The listing builds one solid part. Answer for the finished solid, in the listing's coordinates (mm). Coordinates: 2 decimals unless noted, no trailing zeros. Order: outer loops, then holes, each group sorted by start corner. A loop starts at its lowest first (then second) coordinate and runs counter-clockwise, first axis right, second up. Notation, with made-up numbers: (1.5, 82.5) -> (6.5, 82.5) arc R27 ccw to (6.5, 120.5) -> close; hole circle Ø1 at (-23.5, 41.5). An arc over 180 degrees is marked (long way). Write item = value, one per line. Start each with the question number.
```python
from build123d import *

# Parameters (mm, degrees)
SKETCH_1_R          = 60
EXTRUDE_1_DEPTH     = 2
SKETCH_2_R          = 4
CUT_EXTRUDE_1_DEPTH = 2


with BuildPart() as part:
    # 草图1 → 凸台-拉伸1 (new body)
    with BuildSketch(Plane(origin=(0, 0, 0), x_dir=(1, 0, 0), z_dir=(0, 1, 0))):
        with Locations(Location((0, 0, 0), (0, 0, 270))):
            Circle(SKETCH_1_R)
    extrude(amount=EXTRUDE_1_DEPTH)

    # 草图2 → 切除-拉伸1 (cut)
    with BuildSketch(Plane(origin=(0, 2, 0), x_dir=(1, 0, 0), z_dir=(0, 1, 0))):
        with BuildLine():
            ThreePointArc((-3.5, 5), (-6.060660172, 6.060660172), (-5, 3.5))
            Line((-5, 3.5), (-5, 5))
            Line((-5, 5), (-3.5, 5))
        make_face()
        with BuildLine():
            Line((-5, 5), (-5, 3.5))
            ThreePointArc((-5, 3.5), (-3.939339828, 3.939339828), (-3.5, 5))
            Line((-3.5, 5), (-5, 5))
        make_face()
        with BuildLine():
            ThreePointArc((3.5, 5), (3.939339828, 3.939339828), (5, 3.5))
            Line((5, 3.5), (5, 5))
            Line((5, 5), (3.5, 5))
        make_face()
        with BuildLine():
            Line((5, 5), (5, 3.5))
            ThreePointArc((5, 3.5), (6.060660172, 3.939339828), (6.5, 5))
            ThreePointArc((6.5, 5), (5, 6.5), (3.5, 5))
            Line((3.5, 5), (5, 5))
        make_face()
        with Locations(Location((0, 0, 0), (0, 0, 270))):
            Circle(SKETCH_2_R)
        with BuildLine():
            ThreePointArc((5, -3.5), (3.939339828, -3.939339828), (3.5, -5))
            Line((3.5, -5), (5, -5))
            Line((5, -5), (5, -3.5))
        make_face()
        with BuildLine():
            Line((5, -5), (3.5, -5))
            ThreePointArc((3.5, -5), (5, -6.5), (6.5, -5))
            ThreePointArc((6.5, -5), (6.060660172, -3.939339828), (5, -3.5))
            Line((5, -3.5), (5, -5))
        make_face()
        with BuildLine():
            ThreePointArc((-5, -3.5), (-6.060660172, -6.060660172), (-3.5, -5))
            Line((-3.5, -5), (-5, -5))
            Line((-5, -5), (-5, -3.5))
        make_face()
        with BuildLine():
            Line((-5, -5), (-3.5, -5))
            ThreePointArc((-3.5, -5), (-3.939339828, -3.939339828), (-5, -3.5))
            Line((-5, -3.5), (-5, -5))
        make_face()
    extrude(amount=-CUT_EXTRUDE_1_DEPTH, mode=Mode.SUBTRACT)


solid = part.part
```
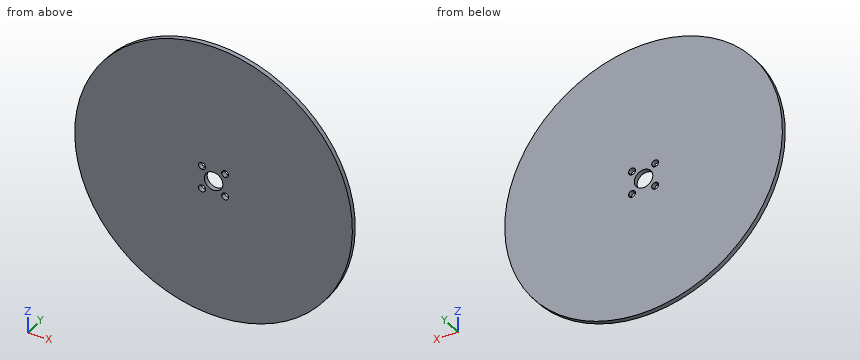
Item 1: Section D-D, the plane z = -41.5 is taken. Give the vertices of the cut face in (x, y).
Item 2: Consider probe 1 along X at (y, z) = (0.65, 0); probe 2 along X at (y, z) = (0.7, -5). Determine where each line is inside the solid, lowest interval first.
Item 3: Section A-A, the plane y = 0.4 is taken. Give the vertices of the cut face in (x, z), then the cut area to 3 significant figures.
Item 4: This flat-tipped pin is pushed along its axis until it touches: pin 1 (1 mm diameter, centred on y = 0.5, z = 47, fed in from -X). Where does it stop, or does it pass through?
Item 5: Section C-C, the plane z = 0 is taken. Give the vertices of the cut face in (x, y).
Item 6: Section B-B, the plane x = 0 is taken. Give the vertices of the cut face in (y, z).
A:
q1.outline = (-43.33, 0) -> (43.33, 0) -> (43.33, 2) -> (-43.33, 2) -> close
q2.probe_1 = -60 to -4, 4 to 60
q2.probe_2 = -59.79 to -6.5, -3.5 to 3.5, 6.5 to 59.79
q3.outline = circle Ø120 at (0, 0); hole circle Ø3 at (-5, -5); hole circle Ø3 at (-5, 5); hole circle Ø8 at (0, 0); hole circle Ø3 at (5, -5); hole circle Ø3 at (5, 5)
q3.area = 11,200 mm^2
q4.pin_1 = -37.92
q5.outline = (-60, 0) -> (-4, 0) -> (-4, 2) -> (-60, 2) -> close; (4, 0) -> (60, 0) -> (60, 2) -> (4, 2) -> close
q6.outline = (0, -60) -> (2, -60) -> (2, -4) -> (0, -4) -> close; (0, 4) -> (2, 4) -> (2, 60) -> (0, 60) -> close
